Design review of the part shown in the three views and the two pictorial views. Dimensions are in mm from the part's minimum x, y and z. A direction names the side the tool comes from. Give positions to 0.01 mm unless a question says otherwise; leave off trailing zeros. Order: outer loops, then holes, each group sorted by start corner. A loop starts at its lowest first (then second) coordinate and runs counter-clockwise, first axis right, second up.
Item 1: For P1, Ø12, axis at y = 18.5, z = 14.5, coming from the +X side; P2, Ø4, axis at x = 10, z = 3, coming from the -Y side; P3, Ø1.5, axis at x = 7, y = 20, coming from the +Z side; P4, Ø5, axis at y = 27, z = 12.5, coming from the -X side, all flat-tipped, find the tip position at first contact; note any pin that passes through.
Item 2: Consider section D-D (y = 22). Give the boundary of the cut face in (x, z).
Item 3: Consider section C-C (x = 10). Give the number of separate pieces and of enclosed holes in the cut face, plus the area to 3 significant figures.
Item 4: For probe 1 along Y at (x, z) = (15, 6.5); probe 2 along X at (y, z) = (15.5, 17.25); probe 3 along X at (y, z) = (19, 17), list the stretches that pass through material, from the lowest coordinate up.
Item 5: Consider section B-B (z = 3.75). Give the boundary of the cut face in (x, y).
Item 6: Consider section A-A (x = 16.75). Give the boundary of the cut face in (y, z), plus the area to 3 significant figures.
Item 7: Machinability: for the marked faces 1, 2 and 3, which of the approach directions +Z, -Z, +X, -X, +Y, -Y give a long, thin tool a straight path to every point of the face, cutting with its end or side? Answer none if there is none.
Item 8: The part is to be moulded in two halves that separate along Z. For the marked faces 4, 5, 6 and 7, say which applies: released by +Z, released by -Z, zero draft, split by the parting line, or undercut.
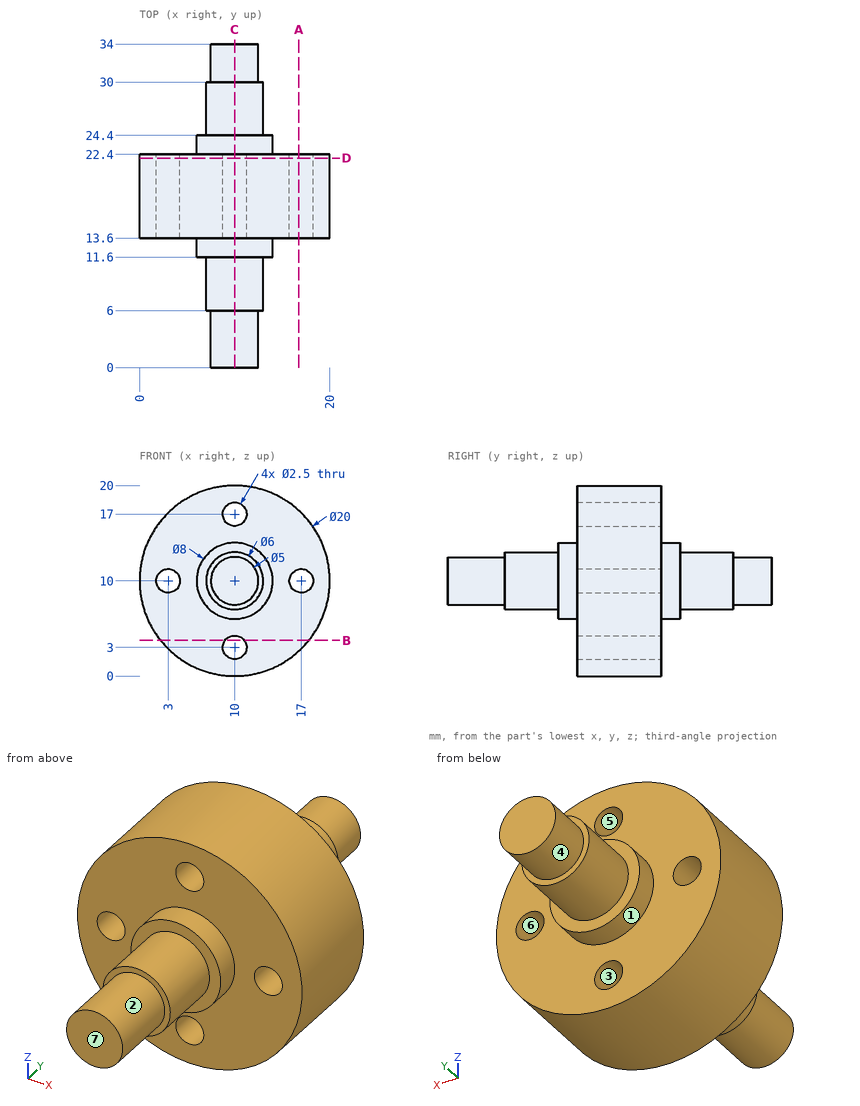
Resolved:
1. P1: stops at x = 20
1. P2: stops at y = 13.6
1. P3: stops at z = 19.74
1. P4: stops at x = 7
2. outline: circle Ø20 at (10, 10); hole circle Ø2.5 at (3, 10); hole circle Ø2.5 at (10, 3); hole circle Ø2.5 at (10, 17); hole circle Ø2.5 at (17, 10)
3. separate pieces: 3
3. enclosed holes: 0
3. area: 281 mm2
4. probe 1: y = 13.6 to 22.4
4. probe 2: x = 3.11 to 8.78, 11.22 to 16.89
4. probe 3: x = 2.86 to 8.75, 11.25 to 17.14
5. outline: (2.19, 13.6) - (9, 13.6) - (9, 22.4) - (2.19, 22.4) - close; (11, 13.6) - (17.81, 13.6) - (17.81, 22.4) - (11, 22.4) - close
6. outline: (13.6, 2.62) - (22.4, 2.62) - (22.4, 8.78) - (13.6, 8.78) - close; (13.6, 11.22) - (22.4, 11.22) - (22.4, 17.38) - (13.6, 17.38) - close
6. area: 108 mm2
7. face 1: +Y
7. face 2: -Y
7. face 3: +Y, -Y
8. face 4: split by the parting line
8. face 5: undercut
8. face 6: undercut
8. face 7: zero draft
